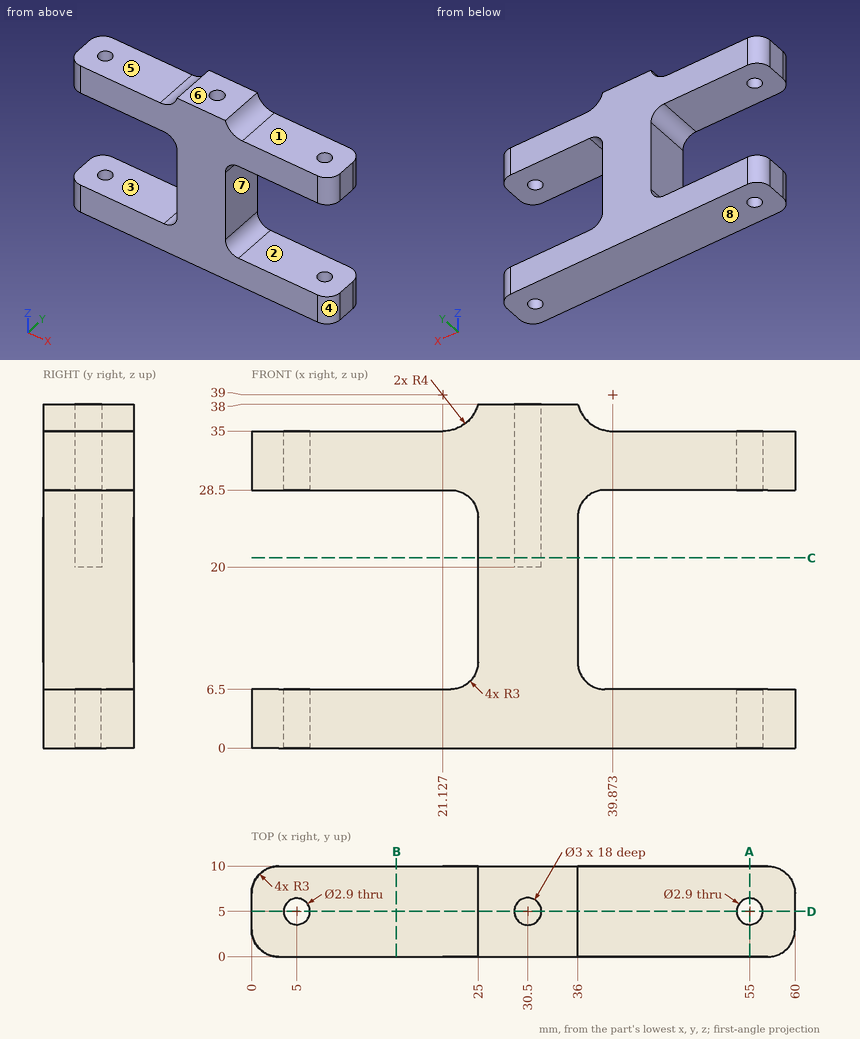
Geometry check sheet. Reference: drawing and pictorial views, mm from the part's lowest x, y, z. A direction names the side the tool comes from. Round coordinates to 2 decimals unless told otherwise and drop trailing zeros. Loops run counter-clockwise (first coordinate to the right, second up) from the corner with the lowest first, then second, coordinate; pieces in that order, holes last. Notation, with made-up numbers: (89.5, 83.25) -> (119.5, 83.25) arc R23 cw to (119.5, 91.25) -> close; hole circle Ø4 at (-17, -39). An arc over 180 degrees is marked (long way). Answer as a JSON object with one key per item and string values.
Q1. Scan lines: line 1 (Z direction, x = 46.5, y = 2); line 2 (Y direction, x = 55, z = 1.75); line 3 (X direction, y = 4, z = 31.5). Record each from-to range of solid material in increasing order. Write a range as from..to.
Data:
{"line 1": "z = 0..6.5, 28.5..35", "line 2": "y = 0..3.55, 6.45..10", "line 3": "x = 0..3.95, 6.05..29.38, 31.62..53.95, 56.05..60"}
Q2. Section check C-C (z = 21). Record the boundary of the cut face in (x, y).
Data:
{"outline": "(25, 0) -> (36, 0) -> (36, 10) -> (25, 10) -> close; hole circle Ø3 at (30.5, 5)"}
Q3. Section check B-B (x = 16). Record the boundary of the cut face in (y, z), then the cut area to 3 significant figures.
Data:
{"outline": "(0, 0) -> (10, 0) -> (10, 6.5) -> (0, 6.5) -> close; (0, 28.5) -> (10, 28.5) -> (10, 35) -> (0, 35) -> close", "area": "130 mm2"}
Q4. Section check D-D (y = 5). State how many separate pieces and enclosed holes the cut face has, then the cut area to 3 significant figures.
Data:
{"separate pieces": "5", "enclosed holes": "0", "area": "939 mm2"}
Q5. Draft check along Z on the marked faces 6, 7 and 8. Enter one of: pulls with the +Z half, pulls with the -Z half, needs draft (parallel to the pull), parting line crosses it, or undercut.
Data:
{"face 6": "pulls with the +Z half", "face 7": "undercut", "face 8": "pulls with the -Z half"}
Q6. Access from +Z, -Z, +X, -X, +Y, -Y to the whole of each face (thin tool, end or side, straight path). Record for the marked faces 1, 2, 3, 4 and 5.
Data:
{"face 1": "+Z, +X, +Y, -Y", "face 2": "+X, +Y, -Y", "face 3": "-X, +Y, -Y", "face 4": "+Z, -Z, +X, -Y", "face 5": "+Z, -X, +Y, -Y"}
Q7. Go/stop test with flat-tipped pins: P1, Ø2.5, axis at x = 30.5, y = 5, coming from the +Z side; P2, Ø3, axis at x = 13, y = 6.5, coming from the +Z side; P3, Ø3, axis at y = 3, z = 20, coming from the +X side. Record where each tip stops, or that it passes through.
Data:
{"P1": "stops at z = 20", "P2": "stops at z = 35", "P3": "stops at x = 36"}
Q8. Section check A-A (x = 55). Record the boundary of the cut face in (y, z).
Data:
{"outline": "(0, 0) -> (3.55, 0) -> (3.55, 6.5) -> (0, 6.5) -> close; (0, 28.5) -> (3.55, 28.5) -> (3.55, 35) -> (0, 35) -> close; (6.45, 0) -> (10, 0) -> (10, 6.5) -> (6.45, 6.5) -> close; (6.45, 28.5) -> (10, 28.5) -> (10, 35) -> (6.45, 35) -> close"}
